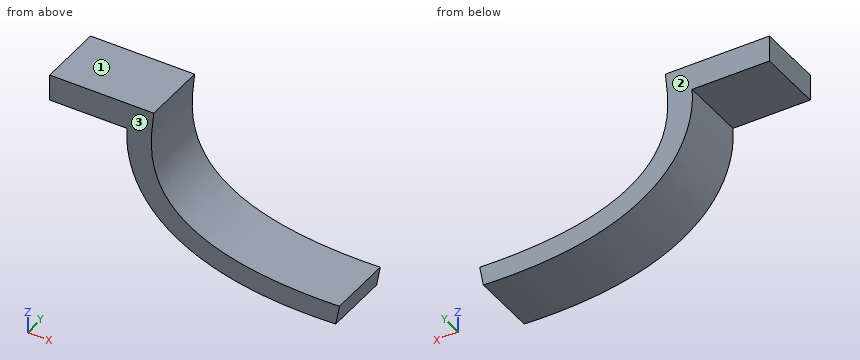
```python
from build123d import *

# Parameters (mm, degrees)
F1_DEPTH = 12.7


with BuildPart() as f1:
    # F0 (on Front) → F1 (new body)
    with BuildSketch(Plane.XZ):
        with BuildLine():
            Line((-31.644711, 35.822344), (-51.697341, 35.822344))
            Line((-51.697341, 35.822344), (-51.697341, 30.742344))
            Line((-51.697341, 30.742344), (-36.811311, 30.742344))
            add(Edge.make_bspline(
                [(-36.811311, 30.742344), (-37.394196, 22.58198), (-33.605456, 4.804045), (3.407622, 6.552694)],
                knots=[0, 0, 0, 0, 46.932949, 46.932949, 46.932949, 46.932949], degree=3))
            Line((3.407622, 6.552694), (4.115814, 10.422344))
            add(Edge.make_bspline(
                [(-31.644711, 35.822344), (-32.313132, 28.469711), (-36.811311, 9.175669), (4.115814, 10.422344)],
                knots=[0, 0, 0, 0, 43.863141, 43.863141, 43.863141, 43.863141], degree=3))
        make_face()
    extrude(amount=-F1_DEPTH)


solid = f1.part
```
For this review, take the finished solid that the model builds, in its own axes (mm). Face numbers are marked on the shaded views. Coordinates: 2 decimals unless noted, no trailing zeros. Write each loop counter-clockwise with the first axis right and the second up, starting at its lowest first coordinate (ties: lowest second). Pieces come first, ordered by that corner, then holes. Notation, with made-up numbers: (26, 46.25) - (70, 46.25) arc R23 cw to (70, 76.25) - close; hole circle Ø6 at (0, 21). An arc over 180 degrees is marked (long way). Answer in a Markdown table with one row per item. Add a question column.
Q1. For probe 1 along Z at (x, y) = (-49, 4.75); probe 2 along Z at (x, y) = (-7, 6.25); probe 3 along X at (y, z) = (3, 32), list the stretches that pass through material, from the lowest coordinate up.
Q2. For P1, Ø4, axis at y = 7, z = 21, coming from the +X side; P2, Ø4, axis at x = -41.5, y = 6.5, coming from the -Z side; P3, Ø2, axis at y = 11, z = 15.5, coming from the +X side; P4, Ø6, axis at x = -31, z = 22.5, coming from the -Y side, all flat-tipped, find the tip position at first contact; note any pin that passes through.
Q3. Draft analysis for pull direction Y (two halves, no side actions). For the marked faces 1, 2 and 3, state which applies: +Y half, -Y half, draft (parallel to the pull), parting line (faces both ways), or undercut.
Q4. We need section A-A, the plane x = -38.5. State the section outline as (y, z) points, and give its area (3 significant figures).
Answer list:
| question | item | result |
|---|---|---|
| 1 | probe 1 | z = 30.74 to 35.82 |
| 1 | probe 2 | z = 6.6 to 10.64 |
| 1 | probe 3 | x = -51.7 to -32.02 |
| 2 | P1 | stops at x = -28.68 |
| 2 | P2 | stops at z = 30.74 |
| 2 | P3 | stops at x = -22.89 |
| 2 | P4 | stops at y = 0 |
| 3 | face 1 | draft |
| 3 | face 2 | +Y half |
| 3 | face 3 | -Y half |
| 4 | outline | (0, 30.74) - (12.7, 30.74) - (12.7, 35.82) - (0, 35.82) - close |
| 4 | area | 64.5 mm2 |
